Source: CAD feature listing. Evaluate the final solid. Frame: model axes, mm. Face numbers are marked on the shaded views. A direction names the side the tool comes from. Round coordinates to 2 decimals unless told otherwise and drop trailing zeros. Order: outer loops, then holes, each group sorted by start corner. A loop starts at its lowest first (then second) coordinate and runs counter-clockwise, first axis right, second up. Notation, with made-up numbers: M -11,-30 L 43,-30 A34 cw 43,9 Z; hole C 12.5,83.25 d3. An arc over 180 degrees is marked long. Answer in a Markdown table with one row per item. Add a question column.
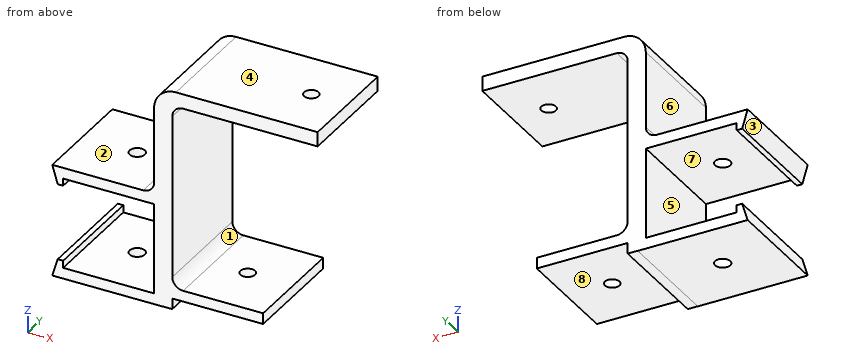
```python
from build123d import *

# Parameters (mm, degrees)
EXTRUDE_1_DEPTH      = 110
CUT_EXTRUDE_4_DEPTH  = 134.373777696
SKETCH_7_W           = 16.60831278
SKETCH_7_H           = 38.473598513
CUT_EXTRUDE_14_DEPTH = 134.373777696
SKETCH_8_W           = 5
SKETCH_8_H           = 30.968526609
EXTRUDE_2_DEPTH      = 110
SKETCH_10_W          = 5
SKETCH_10_H          = 26
EXTRUDE_4_DEPTH      = 110
SKETCH_16_W          = 45
SKETCH_16_H          = 4
EXTRUDE_7_DEPTH      = 110
FILLET_4_R           = 3
FILLET_5_R           = 6
SKETCH_18_W          = 113.67218818
SKETCH_18_H          = 61.649849458
CUT_EXTRUDE_18_DEPTH = 137.586229955
SKETCH_19_R          = 2.1
SKETCH_19_R_2        = 2
CUT_EXTRUDE_19_DEPTH = 143.431323365
SKETCH_22_W          = 25
SKETCH_22_H          = 3
EXTRUDE_10_DEPTH     = 30
FILLET_7_R           = 3
SKETCH_23_R          = 2
CUT_EXTRUDE_24_DEPTH = 10
SKETCH_24_W          = 79.129869038
SKETCH_24_H          = 20.357001259
CUT_EXTRUDE_25_DEPTH = 143.431323365


# Read off the part's stored shape, not the designer's step: Бобышка-Вытянуть1
with BuildPart() as part:
    # Бобышка-Вытянуть1 outline → Бобышка-Вытянуть1 (new body)
    with BuildSketch(Plane(origin=(0, 0, 0), x_dir=(1, 0, 0), z_dir=(0, 1, 0))):
        Polygon((-36.579007505, 34.969739794), (-66.825757576, 34.969739794), (-66.825757576, 29.969739794), (-63.825757576, 29.969739794), (-63.825757576, 31.969739794), (-38.825757576, 31.969739794), (-38.825757576, 6.969739794), (-63.825757576, 6.969739794), (-63.825757576, 8.969739794), (-66.825757576, 8.969739794), (-66.825757576, 3.969739794), (-22.123470102, 3.969739794), align=None)
    extrude(amount=EXTRUDE_1_DEPTH)

    # Эскиз3 → Вырез-Вытянуть4 (cut, through all)
    with BuildSketch(Plane.XZ):
        Polygon((-66.825757576, -3.969739794), (-65.325757576, -8.969739794), (-66.825757576, -8.969739794), align=None)
        Polygon((-66.825757576, -29.969739794), (-66.825757576, -34.969739794), (-65.325757576, -29.969739794), align=None)
    extrude(amount=-CUT_EXTRUDE_4_DEPTH, mode=Mode.SUBTRACT)

    # Эскиз7 → Вырез-Вытянуть14 (cut, through all)
    with BuildSketch(Plane(origin=(0, 0, 0), x_dir=(-1, 0, 0), z_dir=(0, -1, 0))):
        with Locations((27.703474463, 20.539743139)):
            Rectangle(SKETCH_7_W, SKETCH_7_H)
    extrude(amount=-CUT_EXTRUDE_14_DEPTH, mode=Mode.SUBTRACT)

    # Эскиз8 → Бобышка-Вытянуть2 (add)
    with BuildSketch(Plane(origin=(0, 0, 0), x_dir=(-1, 0, 0), z_dir=(0, -1, 0))):
        with Locations((36.298943925, 19.454003098)):
            Rectangle(SKETCH_8_W, SKETCH_8_H)
    extrude(amount=-EXTRUDE_2_DEPTH)

    # Эскиз10 → Бобышка-Вытянуть4 (add)
    with BuildSketch(Plane.XZ):
        with Locations((-36.298943925, 9.030260206)):
            Rectangle(SKETCH_10_W, SKETCH_10_H)
    extrude(amount=-EXTRUDE_4_DEPTH)

    # Эскиз16 → Бобышка-Вытянуть7 (add, through all)
    with BuildSketch(Plane(origin=(0, 110, 0), x_dir=(1, 0, 0), z_dir=(0, 1, 0))):
        with Locations((-16.298943925, -24.030260206)):
            Rectangle(SKETCH_16_W, SKETCH_16_H)
    extrude(amount=-EXTRUDE_7_DEPTH)

    # Скругление4
    fillet_4_edges = [part.edges().sort_by_distance(p)[0] for p in [
        (-38.798943925, 55, -3.969739794),
        (-33.798943925, 55, 22.030260206),
    ]]
    fillet(fillet_4_edges, radius=FILLET_4_R)

    # Скругление5
    fillet_5_edges = [part.edges().sort_by_distance(p)[0] for p in [
        (-38.798943925, 55, 26.030260206),
    ]]
    fillet(fillet_5_edges, radius=FILLET_5_R)

    # Эскиз18 → Вырез-Вытянуть18 (cut, through all)
    with BuildSketch(Plane(origin=(6.201056075, 0, 0), x_dir=(0, 0, -1), z_dir=(1, 0, 0))):
        with Locations((3.709673157, 49.175075271)):
            Rectangle(SKETCH_18_W, SKETCH_18_H)
    extrude(amount=-CUT_EXTRUDE_18_DEPTH, mode=Mode.SUBTRACT)


with BuildPart() as cut_extrude_18_piece_1:
    # of the separate pieces the step leaves, piece 1, a body of its own (cut_extrude_18_pieces)
    add(part.part.solids().sort_by_distance((-38.798943925, 110, 20.030260206))[0])

    # Эскиз19 → Вырез-Вытянуть19 (cut, through all)
    with BuildSketch(Plane(origin=(0, 0, -34.969739794), x_dir=(-1, 0, 0), z_dir=(0, 0, -1))):
        with Locations((51.70238254, 95)):
            Circle(SKETCH_19_R)
        with Locations((3.798943925, 95)):
            Circle(SKETCH_19_R_2)
    extrude(amount=-CUT_EXTRUDE_19_DEPTH, mode=Mode.SUBTRACT)

    # Эскиз22 → Бобышка-Вытянуть10 (add)
    with BuildSketch(Plane.XZ.offset(-80)):
        with Locations((-21.298943925, -30.469739794)):
            Rectangle(SKETCH_22_W, SKETCH_22_H)
    extrude(amount=-EXTRUDE_10_DEPTH)

    # Скругление7
    fillet_7_edges = [cut_extrude_18_piece_1.edges().sort_by_distance(p)[0] for p in [
        (-33.798943925, 95, -28.969739794),
    ]]
    fillet(fillet_7_edges, radius=FILLET_7_R)

    # Эскиз23 → Вырез-Вытянуть24 (cut)
    with BuildSketch(Plane(origin=(0, 0, -31.969739794), x_dir=(-1, 0, 0), z_dir=(0, 0, -1))):
        with Locations((21.298943925, 95)):
            Circle(SKETCH_23_R)
    extrude(amount=-CUT_EXTRUDE_24_DEPTH, mode=Mode.SUBTRACT)


with BuildPart() as cut_extrude_18_piece_2:
    # of the separate pieces the step leaves, piece 2, a body of its own (cut_extrude_18_pieces)
    add(part.part.solids().sort_by_distance((-38.798943925, 18.350150542, -0.969739794))[0])

    # Эскиз24 → Вырез-Вытянуть25 (cut, through all)
    with BuildSketch(Plane(origin=(0, 0, -34.969739794), x_dir=(-1, 0, 0), z_dir=(0, 0, -1))):
        with Locations((27.260823057, 8.171649913)):
            Rectangle(SKETCH_24_W, SKETCH_24_H)
    extrude(amount=-CUT_EXTRUDE_25_DEPTH, mode=Mode.SUBTRACT)


solid = cut_extrude_18_piece_1.part
```
(1) Cut plane D-D (x = -38). Return loops of the section in (y, z).
(2) Pin query (flat end, axial travel): pin 1 (2 mm diameter, centred on x = -7.5, y = 95, fed in from -Z); pin 2 (1.5 mm diameter, centred on x = -57.5, z = -1.5, fed in from -Y); pin 3 (1.2 mm diameter, centred on x = -64.5, y = 100.5, fed in from +Z); pin 4 (3.5 mm diameter, centred on y = 100, z = -34, fed in from +X). Return the tip coordinate at first contact, or that it passes through.
(3) Draft query along X for the marked faces 6, 7 and 8. Return one class per face: +X half, -X half, draft (parallel to the pull), parting line (faces both ways), or undercut.
(4) Cut plane B-B (y = 95). Count the separate pieces of the cut face and the enclosed holes in it, and give its area (3 significant figures).
(5) Cut plane C-C (z = -22). Return loops of the section in (x, y), and give its area (3 significant figures).
(6) Access query for the marked faces 1, 2, 3, 4 and 5. Directions: +Z, -Z, +X, -X, +Y, -Y. A direction counts if a zero-diameter tool reaches every point of the face in a straight line with its end or side. Return the directions, or none.
(7) Line query: line 1 (Z direction, x = -57, y = 98.25); line 2 (Z direction, x = -21, y = 108); line 3 (Z direction, x = -1, y = 108). Output: solid intervals per line, ascending. Write a range as from..to.
Answer list:
| question | item | result |
|---|---|---|
| 1 | outline | M 80,-34.97 L 110,-34.97 L 110,23.02 L 80,23.02 Z |
| 2 | pin 1 | z = 22.03 |
| 2 | pin 2 | through |
| 2 | pin 3 | z = -3.97 |
| 2 | pin 4 | x = -33.8 |
| 3 | face 6 | -X half |
| 3 | face 7 | undercut |
| 3 | face 8 | draft |
| 4 | separate pieces | 5 |
| 4 | enclosed holes | 0 |
| 4 | area | 658 mm² |
| 5 | outline | M -38.83,80 L -33.8,80 L -33.8,110 L -38.83,110 Z |
| 5 | area | 151 mm² |
| 6 | face 1 | +X, +Y, -Y |
| 6 | face 2 | +Z, -X, +Y, -Y |
| 6 | face 3 | -X, +Y, -Y |
| 6 | face 4 | +Z, +X, -X, +Y, -Y |
| 6 | face 5 | +Y, -Y |
| 7 | line 1 | -34.97..-31.97, -6.97..-3.97 |
| 7 | line 2 | -31.97..-28.97, 22.03..26.03 |
| 7 | line 3 | 22.03..26.03 |
